from build123d import *

# Parameters (mm, degrees)
ESQUISSE1_W                  = 50
ESQUISSE1_H                  = 42.3
BOSS_EXTRU_1_DEPTH           = 25.5
ESQUISSE4_R                  = 18.1
ENL_V_MAT_EXTRU_3_DEPTH      = 22.5
ENL_V_MAT_EXTRU_4_DEPTH      = 62.713369702
ENL_V_MAT_EXTRU_4_DEPTH_BACK = 62.713369702
ESQUISSE5_R                  = 11
ESQUISSE6_R                  = 1.625
ENL_V_MAT_EXTRU_5_DEPTH      = 10
BOSS_EXTRU_2_DEPTH           = 77.7
ESQUISSE16_W                 = 3
ESQUISSE16_H                 = 8.332527472
BOSS_EXTRU_4_DEPTH           = 52.2
ESQUISSE17_W                 = 86
ESQUISSE17_H                 = 2.5
BOSS_EXTRU_5_DEPTH           = 77.7
BOSS_EXTRU_7_DEPTH           = 5
BOSS_EXTRU_8_DEPTH           = 12
ESQUISSE22_R                 = 9.525
ENL_V_MAT_EXTRU_6_DEPTH      = 10
R_P_TITION_LIN_AIRE2_COUNT   = 2
R_P_TITION_LIN_AIRE2_PITCH   = 30
ESQUISSE23_R                 = 6.5
ENL_V_MAT_EXTRU_7_DEPTH      = 177.868821447
BOSS_EXTRU_9_DEPTH           = 5
ESQUISSE27_W                 = 44
ESQUISSE27_H                 = 2.5
ENL_V_MAT_EXTRU_9_DEPTH      = 10
ESQUISSE24_R                 = 4.1
ENL_V_MAT_EXTRU_8_DEPTH      = 140.81519946
BOSS_EXTRU_10_DEPTH          = 90


with BuildPart() as part:
    # Esquisse1 → Boss.-Extru.1 (new body)
    with BuildSketch(Plane.XY):
        with Locations((25, 21.15)):
            Rectangle(ESQUISSE1_W, ESQUISSE1_H)
    extrude(amount=BOSS_EXTRU_1_DEPTH)

    # Esquisse4 → Enlèv. mat.-Extru.3 (cut)
    with BuildSketch(Plane.XY):
        with Locations(Location((25, 21.15, 0), (0, 0, 180))):
            Circle(ESQUISSE4_R)
    extrude(amount=ENL_V_MAT_EXTRU_3_DEPTH, mode=Mode.SUBTRACT)

    # Esquisse5 → Enlèv. mat.-Extru.4 (cut, two sides: drawn at the far end of the back side and taken through both)
    with BuildSketch(Plane(origin=(37, 0, 25.5), x_dir=(-1, 0, 0), z_dir=(0, 0, -1)).offset(-ENL_V_MAT_EXTRU_4_DEPTH_BACK)):
        with Locations((12, 21.15)):
            Circle(ESQUISSE5_R)
    extrude(amount=ENL_V_MAT_EXTRU_4_DEPTH + ENL_V_MAT_EXTRU_4_DEPTH_BACK, mode=Mode.SUBTRACT)

    # Esquisse6 → Enlèv. mat.-Extru.5 (cut)
    with BuildSketch(Plane(origin=(0, 0, 25.5), x_dir=(-1, 0, 0), z_dir=(0, 0, -1))):
        with Locations((-34.899494937, 31.049494937)):
            Circle(ESQUISSE6_R)
        with Locations((-15.100505063, 31.049494937)):
            Circle(ESQUISSE6_R)
        with Locations((-15.100505063, 11.250505063)):
            Circle(ESQUISSE6_R)
        with Locations((-34.899494937, 11.250505063)):
            Circle(ESQUISSE6_R)
    extrude(amount=ENL_V_MAT_EXTRU_5_DEPTH, mode=Mode.SUBTRACT)

    # Esquisse7 → Boss.-Extru.2 (add)
    with BuildSketch(Plane.XY.offset(25.5)):
        Polygon((50, 0), (68, 0), (68, 2.5), (52.12286639, 2.5), (50, 8.332527472), align=None)
        Polygon((-18, 0), (-18, 2.5), (-2.12286639, 2.5), (0, 8.332527472), (0, 0), align=None)
    extrude(amount=-BOSS_EXTRU_2_DEPTH)

    # Esquisse16 → Boss.-Extru.4 (add)
    with BuildSketch(Plane(origin=(0, 0, 0), x_dir=(-1, 0, 0), z_dir=(0, 0, -1))):
        with Locations((-1.5, 4.166263736)):
            Rectangle(ESQUISSE16_W, ESQUISSE16_H)
        with Locations((-48.5, 4.166263736)):
            Rectangle(ESQUISSE16_W, ESQUISSE16_H)
    extrude(amount=BOSS_EXTRU_4_DEPTH)

    # Esquisse17 → Boss.-Extru.5 (add)
    with BuildSketch(Plane.XY.offset(25.5)):
        with Locations((25, -1.25)):
            Rectangle(ESQUISSE17_W, ESQUISSE17_H)
    extrude(amount=-BOSS_EXTRU_5_DEPTH)

    # Esquisse20 → Boss.-Extru.7 (add)
    with BuildSketch(Plane.XZ.offset(2.5)):
        Polygon((-18, 25.5), (10, 53.5), (10, 115.5), (40, 115.5), (40, 53.5), (68, 25.5), align=None)
    extrude(amount=-BOSS_EXTRU_7_DEPTH)

    # Esquisse21 → Boss.-Extru.8 (add)
    with BuildSketch(Plane.XY.offset(115.5)):
        with BuildLine():
            Line((10, 2.5), (14, 7.26701437))
            Line((14, 7.26701437), (14, 23.65))
            ThreePointArc((14, 23.65), (25, 34.65), (36, 23.65))
            Line((36, 23.65), (36, 7.26701437))
            Line((36, 7.26701437), (40, 2.5))
            Line((40, 2.5), (10, 2.5))
        make_face()
    boss_extru_8 = extrude(amount=-BOSS_EXTRU_8_DEPTH)

    # Esquisse22 → Enlèv. mat.-Extru.6 (cut)
    with BuildSketch(Plane.XY.offset(115.5)):
        with Locations((25, 21.15)):
            Circle(ESQUISSE22_R)
    enl_v_mat_extru_6 = extrude(amount=-ENL_V_MAT_EXTRU_6_DEPTH, mode=Mode.SUBTRACT)

    # Répétition linéaire2: Boss.-Extru.8, Enlèv. mat.-Extru.6 ×2
    with Locations(*[(0, 0, -i * R_P_TITION_LIN_AIRE2_PITCH) for i in range(1, R_P_TITION_LIN_AIRE2_COUNT)]):
        add(boss_extru_8)
        add(enl_v_mat_extru_6, mode=Mode.SUBTRACT)

    # Esquisse23 → Enlèv. mat.-Extru.7 (cut, through all)
    with BuildSketch(Plane.XY.offset(105.5)):
        with Locations((25, 21.15)):
            Circle(ESQUISSE23_R)
    extrude(amount=-ENL_V_MAT_EXTRU_7_DEPTH, mode=Mode.SUBTRACT)

    # Esquisse26 → Boss.-Extru.9 (add)
    with BuildSketch(Plane.XZ.offset(2.5)):
        Polygon((-18, -52.2), (3.131019852, -88.8), (46.868980148, -88.8), (68, -52.2), align=None)
    extrude(amount=-BOSS_EXTRU_9_DEPTH)

    # Esquisse27 → Enlèv. mat.-Extru.9 (cut)
    with BuildSketch(Plane.XY.offset(-52.2)):
        with Locations((25, 1.25)):
            Rectangle(ESQUISSE27_W, ESQUISSE27_H)
    extrude(amount=-ENL_V_MAT_EXTRU_9_DEPTH, mode=Mode.SUBTRACT)

    # Esquisse24 → Enlèv. mat.-Extru.8 (cut, through all)
    with BuildSketch(Plane(origin=(0, 2.5, 0), x_dir=(1, 0, 0), z_dir=(0, 1, 0))):
        with Locations(Location((61.62286639, -6.45, 0), (0, 0, 180))):
            Circle(ESQUISSE24_R)
        with Locations(Location((-11.62286639, -6.45, 0), (0, 0, 180))):
            Circle(ESQUISSE24_R)
        with Locations(Location((5.95, 69.75, 0), (0, 0, 180))):
            Circle(ESQUISSE24_R)
        with Locations(Location((44.05, 69.75, 0), (0, 0, 180))):
            Circle(ESQUISSE24_R)
    extrude(amount=-ENL_V_MAT_EXTRU_8_DEPTH, mode=Mode.SUBTRACT)

    # Esquisse28 → Boss.-Extru.10 (add)
    with BuildSketch(Plane.XY.offset(115.5)):
        Polygon((14, 7.26701437), (14, 2.5), (10, 2.5), align=None)
        Polygon((36, 7.26701437), (36, 2.5), (40, 2.5), align=None)
    extrude(amount=-BOSS_EXTRU_10_DEPTH)


solid = part.part
Check sheet for the modelled part. Datum: model origin and axes. Units: mm. A direction names the side the tool comes from. Give positions to 0.01 mm unless a question says otherwise; leave off trailing zeros. Write each loop counter-clockwise with the first axis right and the second up, starting at its lowest first coordinate (ties: lowest second). Pieces come first, ordered by that corner, then holes. Notation, with made-up numbers: M -38,-18 L -9,-18 A10 cw -9,-4 Z; hole C 0,-3.5 d7. An arc over 180 degrees is marked long. Use one line per item in the form item = value.
(1) Material ranges on line 1 along Z through (x, y) = (19, 32.5); line 2 along Z through (x, y) = (14.5, 3.5); line 3 along X through (y, z) = (21, 2.5), recorded low to high.
Answer block:
line_1 = 22.5 to 25.5, 73.5 to 85.5, 103.5 to 115.5
line_2 = 0 to 25.5, 73.5 to 85.5, 103.5 to 115.5
line_3 = 0 to 6.9, 43.1 to 50
(2) Depth check by flat-ended pin: P1, Ø13, axis at y = 11.5, z = 110.5, coming from the +X side; P2, Ø13, axis at y = 27, z = 15, coming from the -X side; P3, Ø17.5, axis at x = 27, z = 42, coming from the +Y side; P4, Ø25, axis at x = 25, y = 21.15, coming from the +Z side. Enter the tip coordinate at first touch or a pass-through.
Answer block:
P1 = 37.9
P2 = 0
P3 = 2.5
P4 = 115.5
(3) Draft check along Y on faces 1 (the cylindrical face through (24.758, 34.647, 109.584)), 2 (the flat face through (10, 0, 84)), 3 (the cylindrical face through (14.508, 24.454, 24.021)). Enter one of: pulls with the +Y half, pulls with the -Y half, needs draft (parallel to the pull), parting line crosses it, or undercut.
Answer block:
face_1 = pulls with the +Y half
face_2 = needs draft
face_3 = undercut
(4) Section check B-B on x = 25. State how many separate pieces and enclosed holes the cut face has, plus the area to 3 significant figures.
Answer block:
separate_pieces = 4
enclosed_holes = 0
area = 1,340 mm2
(5) Section check D-D on z = -69.75. Record the boundary of the cut face in (x, y).
Answer block:
outline = M -7.87,-2.5 L 1.85,-2.5 L 1.85,2.5 L -7.87,2.5 Z; M 10.05,-2.5 L 39.95,-2.5 L 39.95,2.5 L 10.05,2.5 Z; M 48.15,-2.5 L 57.87,-2.5 L 57.87,2.5 L 48.15,2.5 Z
(6) Tool access check on faces 4 (the flat face through (27.6, 11.7, 85.5)), 5 (the flat face through (17, 29, 22.5)), 6 (the cylindrical face through (22.94, 11.85, 110.57)). Record the directions out of +Z, -Z, +X, -X, +Y, -Y that give a thin tool (end or side, any length) a straight path to the whole face; none if there is none.
Answer block:
face_4 = +Y
face_5 = -Z
face_6 = +Z
(7) Section check A-A on z = 20. Record the boundary of the cut face in (x, y), plus the area to 3 significant figures.
Answer block:
outline = M -18,-2.5 L 68,-2.5 L 68,2.5 L 52.12,2.5 L 50,8.33 L 50,42.3 L 0,42.3 L 0,8.33 L -2.12,2.5 L -18,2.5 Z; hole C 25,21.15 d36.2
area = 1,400 mm2
